For this review, use the dimensioned drawing (mm, ordinates from the lowest corner) and the shaded views. A direction names the side the tool comes from. Round coordinates to 2 decimals unless told otherwise and drop trailing zeros. Loops run counter-clockwise (first coordinate to the right, second up) from the corner with the lowest first, then second, coordinate; pieces in that order, holes last. Notation, with made-up numbers: (70, 7) -> (102, 7) arc R8 ccw to (102, 20) -> close; hole circle Ø11 at (-21.75, 22.25). An arc over 180 degrees is marked (long way). Write each question's results on one line, items separated by ' | '.
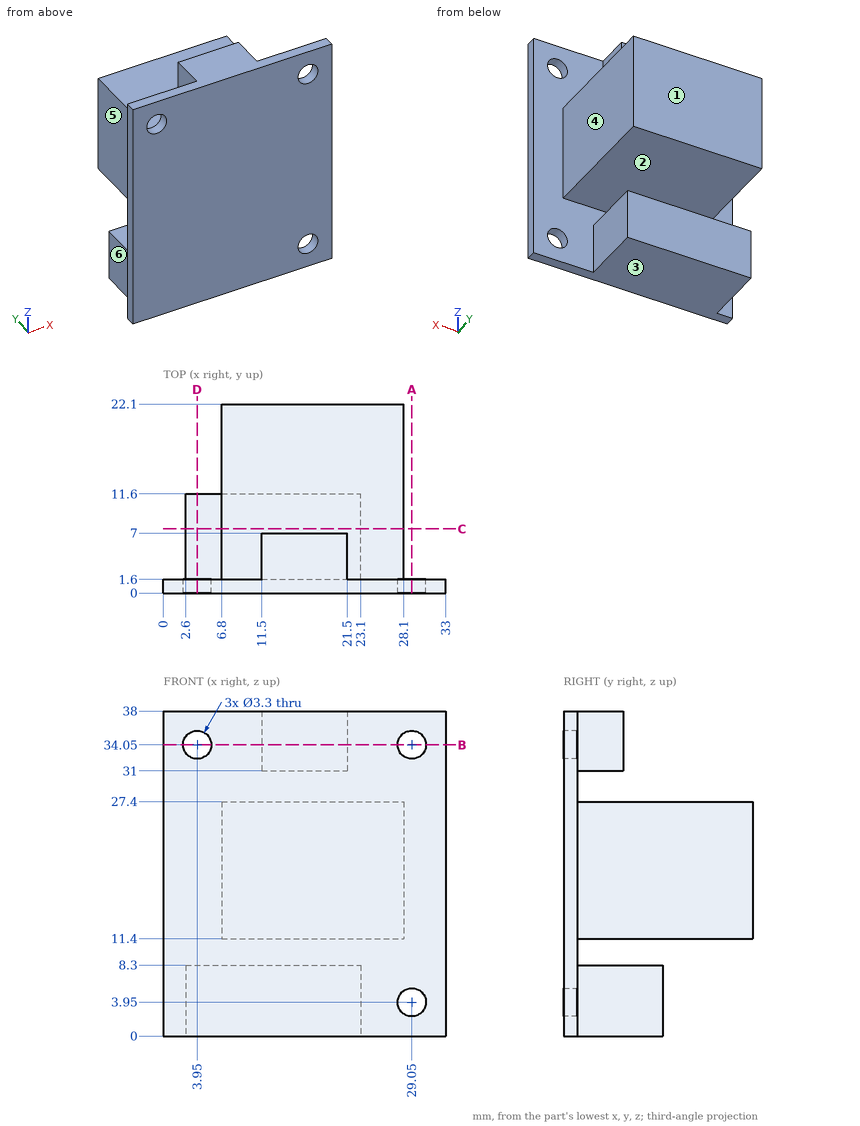
1. Consider section C-C (y = 7.5). State the section outline as (x, z) points, plus the area to 3 significant figures.
Values found:
outline: (2.6, 0) -> (23.1, 0) -> (23.1, 8.3) -> (2.6, 8.3) -> close; (6.8, 11.4) -> (28.1, 11.4) -> (28.1, 27.4) -> (6.8, 27.4) -> close | area: 511 mm2
2. Draft analysis for pull direction Z (two halves, no side actions). For the marked faces 1, 2 and 3, state which applies: released by +Z, released by -Z, zero draft, split by the parting line, or undercut.
Values found:
face 1: zero draft | face 2: undercut | face 3: released by -Z
3. Consider section B-B (z = 34.05). State the section outline as (x, y) points, plus the area to 3 significant figures.
Values found:
outline: (0, 0) -> (2.3, 0) -> (2.3, 1.6) -> (0, 1.6) -> close; (5.6, 0) -> (27.4, 0) -> (27.4, 1.6) -> (21.5, 1.6) -> (21.5, 7) -> (11.5, 7) -> (11.5, 1.6) -> (5.6, 1.6) -> close; (30.7, 0) -> (33, 0) -> (33, 1.6) -> (30.7, 1.6) -> close | area: 96.2 mm2
4. Consider section D-D (x = 3.95). State the section outline as (y, z) points, plus the area to 3 significant figures.
Values found:
outline: (0, 0) -> (11.6, 0) -> (11.6, 8.3) -> (1.6, 8.3) -> (1.6, 32.4) -> (0, 32.4) -> close; (0, 35.7) -> (1.6, 35.7) -> (1.6, 38) -> (0, 38) -> close | area: 139 mm2
5. Tool access review of the marked faces 4, 5 and 6: name each direction out of +Z, -Z, +X, -X, +Y, -Y from which nothing blocks a thin tool from reaching the whole face with its end or side.
Values found:
face 4: +Z, -Z, +X, +Y | face 5: +Z, -X, +Y | face 6: +Z, -Z, -X, +Y
6. Consider section A-A (x = 29.05). State the section outline as (y, z) points, plus the area to 3 significant figures.
Values found:
outline: (0, 0) -> (1.6, 0) -> (1.6, 2.3) -> (0, 2.3) -> close; (0, 5.6) -> (1.6, 5.6) -> (1.6, 32.4) -> (0, 32.4) -> close; (0, 35.7) -> (1.6, 35.7) -> (1.6, 38) -> (0, 38) -> close | area: 50.2 mm2
7. To check wall thickness, follow probe 1 along X at (y, z) = (1.35, 34.05); probe 2 along Z at (x, y) = (21, 7.75); probe 3 along Y at (x, z) = (20.5, 3.5). State the ranges of each line that lie inside material, in increasing order.
Values found:
probe 1: x = 0 to 2.3, 5.6 to 27.4, 30.7 to 33 | probe 2: z = 0 to 8.3, 11.4 to 27.4 | probe 3: y = 0 to 11.6
8. For pin 1 (8 mm diameter, centred on y = 10.5, z = 18.5, fed in from +X); pin 2 (2.5 mm diameter, centred on y = 4.5, z = 33, fed in from -X); pin 3 (7.5 mm diameter, centred on x = 16, z = 36, fed in from +Y); pin 4 (6 mm diameter, centred on x = 13.5, y = 14.5, fed in from -Z), all flat-tipped, find the tip position at first contact; note any pin that passes through.
Values found:
pin 1: stops at x = 28.1 | pin 2: stops at x = 11.5 | pin 3: stops at y = 7 | pin 4: stops at z = 0
